```python
from build123d import *

# Parameters (mm, degrees)
F0_W     = 38.5
F0_H     = 38.5
F1_DEPTH = 1
F0_W_2   = 40.5
F0_H_2   = 40.5
F2_DEPTH = 15
F3_R     = 5


with BuildPart() as f1:
    # F0 (on Top) → F1 (new body)
    with BuildSketch(Plane.XY):
        Rectangle(F0_W, F0_H)
    extrude(amount=F1_DEPTH)

    # F0 (on Top) → F2 (join)
    with BuildSketch(Plane.XY):
        Rectangle(F0_W_2, F0_H_2)
        Rectangle(F0_W, F0_H, mode=Mode.SUBTRACT)
    extrude(amount=F2_DEPTH)

    # F3
    f3_edges = [f1.edges().sort_by_distance(p)[0] for p in [
        (20.25, -20.25, 7.5),
        (19.25, -19.25, 8),
        (-19.25, -19.25, 8),
        (-19.25, 19.25, 8),
        (19.25, 19.25, 8),
        (-20.25, -20.25, 7.5),
        (-20.25, 20.25, 7.5),
        (20.25, 20.25, 7.5),
    ]]
    fillet(f3_edges, radius=F3_R)


solid = f1.part
```
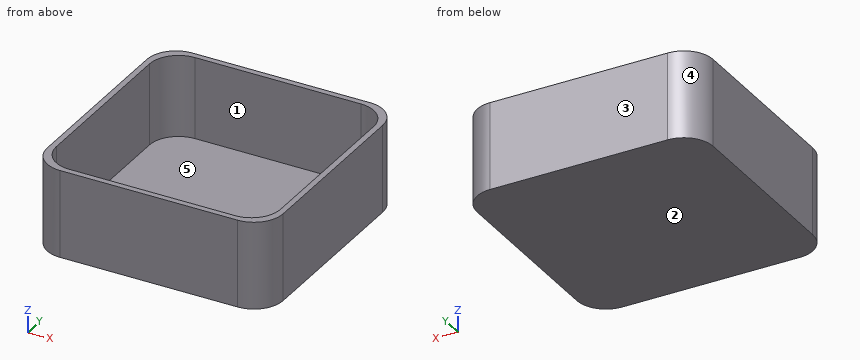
Input: part model. Units: mm. Frame: model coordinates. Face numbers are marked on the shaded views. A direction names the side the tool comes from. Round coordinates to 2 decimals unless told otherwise and drop trailing zeros. Write each loop counter-clockwise with the first axis right and the second up, starting at its lowest first coordinate (ties: lowest second). Pieces come first, ordered by that corner, then holes. Notation, with made-up numbers: M -13,-6 L 36,-6 A22 ccw 36,2 Z; hole C -4.5,82 d8. An arc over 180 degrees is marked long. Write each question's results on one line, items separated by ' | '.
Q1. Section query A-A (z = 3.5). Return loops of the section in (x, y), and give its area (3 significant figures).
Results:
outline: M -20.25,-15.25 A5 ccw -15.25,-20.25 L 15.25,-20.25 A5 ccw 20.25,-15.25 L 20.25,15.25 A5 ccw 15.25,20.25 L -15.25,20.25 A5 ccw -20.25,15.25 Z; hole M -19.25,-14.25 A5 ccw -14.25,-19.25 L 14.25,-19.25 A5 ccw 19.25,-14.25 L 19.25,14.25 A5 ccw 14.25,19.25 L -14.25,19.25 A5 ccw -19.25,14.25 Z | area: 158 mm^2
Q2. Pin query (flat end, axial travel): P1, Ø4, axis at x = -15.5, z = 5, coming from the -Y side; P2, Ø19, axis at x = -4, y = -7.5, coming from the +Z side. Return the tip coordinate at first contact, or that it passes through.
Results:
P1: stops at y = -20.25 | P2: stops at z = 1
Q3. Line query: line 1 along Y through (x, z) = (0.5, 3.25); line 2 along Z through (x, y) = (18.5, 7). Output: solid intervals per line, ascending.
Results:
line 1: y = -20.25 to -19.25, 19.25 to 20.25 | line 2: z = 0 to 1
Q4. Access query for the marked faces 1 and 2. Directions: +Z, -Z, +X, -X, +Y, -Y. A direction counts if a zero-diameter tool reaches every point of the face in a straight line with its end or side. Return the directions, or none.
Results:
face 1: +Z | face 2: -Z, +X, -X, +Y, -Y
Q5. Section query B-B (y = -4.5). Return loops of the section in (x, z), and give its area (3 significant figures).
Results:
outline: M -20.25,0 L 20.25,0 L 20.25,15 L 19.25,15 L 19.25,1 L -19.25,1 L -19.25,15 L -20.25,15 Z | area: 68.5 mm^2
Q6. Draft query along X for the marked faces 3, 4 and 5. Return one class per face: released by +X, released by -X, zero draft, split by the parting line, or undercut.
Results:
face 3: zero draft | face 4: released by -X | face 5: undercut
